Autodesk Inventor part; units mm, degrees
ref_plane "YZ Plane" through (0, 0, 0) normal (1, 0, 0) x (0, 1, 0)
ref_plane "XZ Plane" through (0, 0, 0) normal (0, 1, 0) x (-1, 0, 0)
ref_plane "XY Plane" through (0, 0, 0) normal (0, 0, 1) x (1, 0, 0)
sketch "Szkic1" plane through (0, 0, 0) normal (0, 0, 1) x (1, 0, 0)
  line L0 (-3.8776, -15.6139) -> (12.1224, -15.6139)
  line L1 (12.1224, -15.6139) -> (12.1224, 24.3861)
  line L2 (-3.8776, -15.6139) -> (-3.8776, 24.3861)
  line L3 (-3.8776, 24.3861) -> (12.1224, 24.3861)
  circle A0 centre (4.1224, -7.6139) radius 5.075
  circle A1 centre (4.1224, -7.6139) radius 1.625
  point P0 (0, 0)
  dimension "d0" = 16
  dimension "d1" = 40
  dimension "d2" = 8
  dimension "d3" = 10.15
  dimension "d4" = 8
  dimension "d8" = 3.25
extrude "Wyciągnięcie proste1" add sketch "Szkic1" along normal blind 11 contours L2 L3 L1 L0 | A0
fillet "Zaokrąglenie1" radius 8 2 edges at (-3.8776, -15.6139, 5.5) (12.1224, -15.6139, 5.5)
sketch "Szkic2" plane through (0, 0, 0) normal (0, 0, -1) x (-1, 0, 0)
  arc A0 (-12.1224, -7.6139) -> (3.8776, -7.6139) centre (-4.1224, -7.6139) ccw
  line L0 (-4.1224, -15.6139) -> (-13.9839, -15.6139)
  line L1 (3.8776, 24.3861) -> (3.8776, -7.6139)
  circle A1 centre (-9.1224, 10.3861) radius 2.5
  arc A2 (-12.1224, 14.3861) -> (-12.1224, 6.3861) centre (-9.1224, 10.3861) ccw
  arc A3 (-12.1224, -7.6139) -> (3.8776, -7.6139) centre (-4.1224, -7.6139) ccw
  line L2 (3.8776, 24.3861) -> (3.8776, -7.6139)
  line L3 (-12.1224, 24.3861) -> (3.8776, 24.3861)
  line L4 (-12.1224, -7.6139) -> (-12.1224, 24.3861)
  line L5 (-12.1224, -7.6139) -> (-12.1224, 24.3861)
  line L6 (-12.1224, 19.2527) -> (-8.1224, 19.2527)
  line L7 (-8.1224, 19.2527) -> (-8.1224, 24.3861)
  line L8 (-12.1224, 24.3861) -> (3.8776, 24.3861)
  point P0 (0, 0)
  dimension "d10" = 26
  dimension "d13" = 5
  dimension "d14" = 10
  dimension "d16" = 4
  dimension "d23" = 13
extrude "Wyciągnięcie proste2" add sketch "Szkic2" against normal blind 11 contours A2 L4
extrude "Wyciągnięcie proste3" cut sketch "Szkic2" against normal blind 11.5 contours L4 L3 L7 L6
extrude "Wyciągnięcie proste4" cut sketch "Szkic2" against normal blind 11.5 contours A1
sketch "Szkic3" plane through (-3.8776, 24.3861, 0) normal (-1, 0, 0) x (0, 0, 1)
  line L0 (11, -32) -> (0, -32)
  line L1 (11, 0) -> (11, -32)
  line L2 (0, 0) -> (11, 0)
  line L3 (0, 0) -> (0, -32)
  line L4 (1.75, -23) -> (9.25, -23)
  line L5 (1.75, -23) -> (1.75, -5)
  line L6 (1.75, -5) -> (9.25, -5)
  line L7 (9.25, -5) -> (9.25, -23)
  point P0 (0, -24.3861)
  point P1 (5.75, -14)
  dimension "d24" = 14
  dimension "d26" = 9
  dimension "d27" = 7.5
  dimension "d28" = 11
  dimension "d29" = 18
  dimension "d30" = 1.75
extrude "Wyciągnięcie proste5" cut sketch "Szkic3" against normal blind 20 contours L5 L6 L7 L4
chamfer "Faza3" distance 1.5 distance2 5.1 1 edges at (8.1224, 24.3861, 5.5)
sketch "Szkic5" plane through (0, 0, 0) normal (0, 0, -1) x (-1, 0, 0)
  circle A0 centre (-4.1224, -7.6139) radius 1.625
  circle A1 centre (-4.1224, -7.6139) radius 5.125
  circle A2 centre (-4.1224, -7.6139) radius 2.75
  point P0 (0, 0)
  dimension "d45" = 10.25
  dimension "d64" = 5.5
extrude "Wyciągnięcie proste7" cut sketch "Szkic5" against normal blind 4.1 contours A1 | A2
sketch "Szkic6" plane through (0, 0, 11) normal (0, 0, 1) x (1, 0, 0)
  circle A0 centre (4.1224, -7.6139) radius 5.125
  circle A1 centre (4.1224, -7.6139) radius 1.625
  circle A2 centre (4.1224, -7.6139) radius 2.75
  point P0 (0, 0)
  dimension "d67" = 5.5
extrude "Wyciągnięcie proste8" cut sketch "Szkic6" against normal blind 4.1 contours A0 | A2
sketch "Szkic7" plane through (0, 0, 0) normal (0, 0, -1) x (-1, 0, 0)
  circle A0 centre (-4.1224, -7.6139) radius 5.125
  line L0 (-8.1224, 19.2861) -> (-6.6224, 24.3861)
  line L1 (-8.1224, 19.2861) -> (-8.1224, 19.2527)
  line L2 (-12.1224, 14.3861) -> (-12.1224, 19.2527)
  arc A1 (-12.1224, 14.3861) -> (-12.1224, 6.3861) centre (-9.1224, 10.3861) ccw
  arc A2 (-12.1224, -7.6139) -> (3.8776, -7.6139) centre (-4.1224, -7.6139) ccw
  line L3 (3.8776, 24.3861) -> (3.8776, -7.6139)
  line L4 (-6.6224, 24.3861) -> (3.8776, 24.3861)
  circle A3 centre (-9.1224, 10.3861) radius 2.5
  line L5 (-6.6224, 24.3861) -> (-6.6224, 37.8861)
  line L6 (-0.8724, 24.3861) -> (-0.8724, 34.8861)
  line L7 (-0.8724, 34.8861) -> (3.8776, 34.8861)
  line L8 (3.8776, 34.8861) -> (3.8776, 37.8861)
  line L9 (3.8776, 37.8861) -> (-6.6224, 37.8861)
  line L10 (-8.1224, 19.2527) -> (-12.1224, 19.2527)
  line L11 (-12.1224, -7.6139) -> (-12.1224, 6.3861)
  point P0 (0, 0)
  dimension "d50" = 13.5
  dimension "d52" = 5.75
  dimension "d53" = 10.5
extrude "Wyciągnięcie proste9" add sketch "Szkic7" against normal blind 11 contours L5 L9 L8 L7 L6 L4
fillet "Zaokrąglenie2" radius 2 1 edges at (6.6224, 37.8861, 5.5)
chamfer "Faza4" distance 4.8 distance2 4 1 edges at (12.1224, 19.2527, 0.875) measured on face at (12.1224, 16.0083, 0.5833)
chamfer "Faza5" distance 4.8 distance2 4 1 edges at (12.1224, 19.2527, 10.125) measured on face at (12.1224, 16.0083, 9.8333)
extrude "Wyciągnięcie proste10" cut sketch "Szkic5" against normal blind 4.3 contours A2
extrude "Wyciągnięcie proste11" cut sketch "Szkic6" against normal blind 4.3 contours A2
sketch "Szkic9" plane through (0.8724, 24.3861, 0) normal (-1, 0, 0) x (0, 0, 1)
  line L0 (0, 0) -> (0, 10.5)
  line L1 (11, 0) -> (0, 0)
  line L2 (11, 10.5) -> (11, 0)
  line L3 (0, 10.5) -> (11, 10.5)
  point P0 (0, -24.3861)
  point P1 (5.5, 5.25)
  dimension "d73" = 5.5
  dimension "d74" = 11
  dimension "d75" = 5.25
  dimension "d76" = 10.5
hole "Otwór1" at (0.8724, 29.6361, 5.5) direction (1, 0, 0) diameter 3.25 end through all
sketch "Szkic10" plane through (6.6224, 24.3861, 11) normal (1, 0, 0) x (0, 0, -1)
  circle A0 centre (5.5, 5.25) radius 1.625
  line L0 (0, 11.5) -> (11, 11.5)
  line L1 (0, 0) -> (0, 11.5)
  line L2 (11, 0) -> (0, 0)
  line L3 (11, 11.5) -> (11, 0)
  line L4 (8.4, 3.5757) -> (5.5, 1.9014)
  line L5 (5.5, 1.9014) -> (2.6, 3.5757)
  line L6 (2.6, 3.5757) -> (2.6, 6.9243)
  line L7 (2.6, 6.9243) -> (5.5, 8.5986)
  line L8 (5.5, 8.5986) -> (8.4, 6.9243)
  line L9 (8.4, 6.9243) -> (8.4, 3.5757)
  point P0 (11, -24.3861)
  point P1 (8.4, 5.25)
extrude "Wyciągnięcie proste13" cut sketch "Szkic10" against normal blind 2 contours L4 L5 L6 L7 L8 L9
chamfer "Faza6" distance 5 distance2 3.2 1 edges at (12.1224, 6.3861, 0.875)
chamfer "Faza7" [suppressed]
equation "\"d30\" = -0.5 * d27 + 0.5 * d28"
properties part number "3DP_ABS_Extruder_Tensioning_Arm"
Source: CAD feature listing. Evaluate the final solid. Frame: model axes, mm. A direction names the side the tool comes from. Round coordinates to 2 decimals unless told otherwise and drop trailing zeros. Loops run counter-clockwise (first coordinate to the right, second up) from the corner with the lowest first, then second, coordinate; pieces in that order, holes last. Notation, with made-up numbers: M 44.5,10.5 L 98.5,10.5 A34 cw 98.5,41.5 Z; hole C 43.5,-21 d5. An arc over 180 degrees is marked long. Return JSON: item names as keys, results as strings. Group by question number.
1. Material intervals for line 1 along Z through (x, y) = (2.5, 2); line 2 along Y through (x, z) = (-1, 4.75); line 3 along Y through (x, z) = (5.5, 5.5), sorted ascending. Write a range as from..to.
2. Section query C-C on y = 13.5. Output: boundary loops of the cut face in (x, z), and give its area (3 significant figures).
3. Section query A-A on x = 9.75. Output: boundary loops of the cut face in (y, z), and give its area (3 significant figures).
4. Pin query (flat end, axial travel): pin 1 (5 mm diameter, centred on x = 5.5, y = -6.5, fed in from +Z); pin 2 (3 mm diameter, centred on y = 25.5, z = 9, fed in from +X); pin 3 (7 mm diameter, centred on x = 4.12, y = -7.61, fed in from -Z); pin 4 (4 mm diameter, centred on x = 9.12, y = 10.39, fed in from -Z). Return the tip coordinate at first contact, or that it passes through.
5. Section query D-D on y = -1.5. Output: boundary loops of the cut face in (x, z), and give its area (3 significant figures).
6. Mould query, pull axis X, two halves, no side actions, for faces 1 (the face through (5.636, 27.136, 4.03)), 2 (the face through (13.846, 12.026, 10.113)), 3 (the face through (-0.766, -6.074, 2.021)). Classes: released by +X, released by -X, zero draft, split by the parting line, or undercut.
7. Reachability of faces 4 (the face through (3, 10, 1.75)), 5 (the face through (6, -10, 6.9)), 6 (the face through (5.64, 32.16, 4.07)) from +Z, -Z, +X, -X, +Y, -Y: full face, straight path, thin tool, end or side. Return the list, or none.
8. Section query B-B on z = 10. State how many separate pieces and enclosed holes the cut face has, and give its area (3 significant figures).
Checks:
{
 "1": {"line 1": "z = 0..1.75, 9.25..11", "line 2": "y = -13.76..1.39, 19.39..24.39, 34.89..37.89", "line 3": "y = -15.49..-8.48, -6.75..1.39, 19.39..26.29, 32.98..37.68"},
 "2": {"outline": "M -3.88,0 L 13.03,0 L 13.03,1.75 L -3.88,1.75 Z; M -3.88,9.25 L 13.03,9.25 L 13.03,11 L -3.88,11 Z", "area": "59.2 mm²"},
 "3": {"outline": "M -13.3,0 L 7.97,0 L 7.97,1.75 L 1.39,1.75 L 1.39,9.25 L 7.97,9.25 L 7.97,11 L -13.3,11 Z; M 12.81,0 L 17.3,0 L 17.3,1.75 L 12.81,1.75 Z; M 12.81,9.25 L 17.3,9.25 L 17.3,11 L 12.81,11 Z", "area": "200 mm²"},
 "4": {"pin 1": "stops at z = 6.9", "pin 2": "stops at x = 6.74", "pin 3": "stops at z = 4.1", "pin 4": "passes through"},
 "5": {"outline": "M -3.88,0 L 12.12,0 L 12.12,11 L -3.88,11 Z", "area": "176 mm²"},
 "6": {"face 1": "zero draft", "face 2": "released by +X", "face 3": "undercut"},
 "7": {"face 4": "+X, -X", "face 5": "+Z", "face 6": "+X"},
 "8": {"separate pieces": "1", "enclosed holes": "2", "area": "583 mm²"}
}
